Design review of the part built by this model. Coordinates are the model's own, in mm. A direction names the side the tool comes from. Give positions to 0.01 mm unless a question says otherwise; leave off trailing zeros. Loops run counter-clockwise (first coordinate to the right, second up) from the corner with the lowest first, then second, coordinate; pieces in that order, holes last. Notation, with made-up numbers: (63, -22) - (112, -22) arc R31 ccw to (112, 16) - close; hole circle Ø11 at (81, 79). An arc over 180 degrees is marked (long way). Write each question's results on one line, items separated by ' | '.
```python
from build123d import *

# Parameters (mm, degrees)
SKETCH1_W                       = 533.4
SKETCH1_H                       = 2413
BOSS_EXTRUDE1_DEPTH             = 6.35
F_5_16_0_3125_DIAMETER_HOLE1_D  = 7.9375
F_1_4_0_25_DIAMETER_SLOT1_DEPTH = 6.35


# Read off the part's stored shape, not the designer's step: 1/4 (0.25) Diameter Slot1
with BuildPart() as part:
    # Sketch1 → Boss-Extrude1 (new body)
    with BuildSketch(Plane.XY):
        with Locations((0, 1206.5)):
            Rectangle(SKETCH1_W, SKETCH1_H)
        with BuildLine():
            Line((-101.6, 797.56), (101.6, 797.56))
            Line((101.6, 797.56), (101.6, 663.332045059))
            ThreePointArc((101.6, 663.332045059), (209.55, 480.06), (101.6, 296.787954941))
            Line((101.6, 296.787954941), (101.6, 162.56))
            Line((101.6, 162.56), (-101.6, 162.56))
            Line((-101.6, 162.56), (-101.6, 296.787954941))
            ThreePointArc((-101.6, 296.787954941), (-209.55, 480.06), (-101.6, 663.332045059))
            Line((-101.6, 663.332045059), (-101.6, 797.56))
        make_face(mode=Mode.SUBTRACT)
        with BuildLine():
            Line((-101.6, 1508.76), (-101.6, 1374.532045059))
            ThreePointArc((-101.6, 1374.532045059), (-209.55, 1191.26), (-101.6, 1007.987954941))
            Line((-101.6, 1007.987954941), (-101.6, 873.76))
            Line((-101.6, 873.76), (101.6, 873.76))
            Line((101.6, 873.76), (101.6, 1007.987954941))
            ThreePointArc((101.6, 1007.987954941), (209.55, 1191.26), (101.6, 1374.532045059))
            Line((101.6, 1374.532045059), (101.6, 1508.76))
            Line((101.6, 1508.76), (-101.6, 1508.76))
        make_face(mode=Mode.SUBTRACT)
        with BuildLine():
            Line((-101.6, 2219.96), (-101.6, 2085.732045059))
            ThreePointArc((-101.6, 2085.732045059), (-209.55, 1902.46), (-101.6, 1719.187954941))
            Line((-101.6, 1719.187954941), (-101.6, 1584.96))
            Line((-101.6, 1584.96), (101.6, 1584.96))
            Line((101.6, 1584.96), (101.6, 1719.187954941))
            ThreePointArc((101.6, 1719.187954941), (209.55, 1902.46), (101.6, 2085.732045059))
            Line((101.6, 2085.732045059), (101.6, 2219.96))
            Line((101.6, 2219.96), (-101.6, 2219.96))
        make_face(mode=Mode.SUBTRACT)
    extrude(amount=BOSS_EXTRUDE1_DEPTH)

    # 5/16 (0.3125) Diameter Hole1 (through all)
    with Locations(Plane.XY.offset(6.35)):
        with Locations((-76.2, 146.685), (-76.2, 102.235), (-228.6, 177.8), (76.2, 102.235), (76.2, 146.685), (-76.2, 857.885), (-76.2, 813.435), (76.2, 813.435), (76.2, 857.885), (-76.2, 1569.085), (-76.2, 1524.635), (76.2, 1524.635), (76.2, 1569.085), (-76.2, 2280.285), (-76.2, 2235.835), (76.2, 2235.835), (76.2, 2280.285), (228.6, 177.8), (-228.6, 889), (228.6, 889), (-228.6, 1600.2), (228.6, 1600.2), (-228.6, 2311.4), (228.6, 2311.4)):
            Hole(F_5_16_0_3125_DIAMETER_HOLE1_D / 2)

    # 1/4 (0.25) Diameter Slot1 outline → 1/4 (0.25) Diameter Slot1 (cut)
    with BuildSketch(Plane.XY):
        with BuildLine():
            Line((135.8265, 2182.569545059), (135.8265, 2122.244545059))
            ThreePointArc((135.8265, 2122.244545059), (139.0015, 2119.069545059), (142.1765, 2122.244545059))
            Line((142.1765, 2122.244545059), (142.1765, 2182.569545059))
            ThreePointArc((142.1765, 2182.569545059), (139.0015, 2185.744545059), (135.8265, 2182.569545059))
        make_face()
        with BuildLine():
            Line((142.1765, 1411.044545059), (142.1765, 1471.369545059))
            ThreePointArc((142.1765, 1471.369545059), (139.0015, 1474.544545059), (135.8265, 1471.369545059))
            Line((135.8265, 1471.369545059), (135.8265, 1411.044545059))
            ThreePointArc((135.8265, 1411.044545059), (139.0015, 1407.869545059), (142.1765, 1411.044545059))
        make_face()
        with BuildLine():
            Line((142.1765, 699.844545059), (142.1765, 760.169545059))
            ThreePointArc((142.1765, 760.169545059), (139.0015, 763.344545059), (135.8265, 760.169545059))
            Line((135.8265, 760.169545059), (135.8265, 699.844545059))
            ThreePointArc((135.8265, 699.844545059), (139.0015, 696.669545059), (142.1765, 699.844545059))
        make_face()
        with BuildLine():
            Line((-142.1765, 2182.569545059), (-142.1765, 2122.244545059))
            ThreePointArc((-142.1765, 2122.244545059), (-139.0015, 2119.069545059), (-135.8265, 2122.244545059))
            Line((-135.8265, 2122.244545059), (-135.8265, 2182.569545059))
            ThreePointArc((-135.8265, 2182.569545059), (-139.0015, 2185.744545059), (-142.1765, 2182.569545059))
        make_face()
        with BuildLine():
            Line((-135.8265, 1411.044545059), (-135.8265, 1471.369545059))
            ThreePointArc((-135.8265, 1471.369545059), (-139.0015, 1474.544545059), (-142.1765, 1471.369545059))
            Line((-142.1765, 1471.369545059), (-142.1765, 1411.044545059))
            ThreePointArc((-142.1765, 1411.044545059), (-139.0015, 1407.869545059), (-135.8265, 1411.044545059))
        make_face()
        with BuildLine():
            Line((-135.8265, 699.844545059), (-135.8265, 760.169545059))
            ThreePointArc((-135.8265, 760.169545059), (-139.0015, 763.344545059), (-142.1765, 760.169545059))
            Line((-142.1765, 760.169545059), (-142.1765, 699.844545059))
            ThreePointArc((-142.1765, 699.844545059), (-139.0015, 696.669545059), (-135.8265, 699.844545059))
        make_face()
    extrude(amount=F_1_4_0_25_DIAMETER_SLOT1_DEPTH, mode=Mode.SUBTRACT)


solid = part.part
```
Item 1: We need section C-C on y = 1839. Give the boundary of the cut face in (x, z), then the cut area to 3 significant figures.
Output values:
outline: (-266.7, 0) - (-199.71, 0) - (-199.71, 6.35) - (-266.7, 6.35) - close; (199.71, 0) - (266.7, 0) - (266.7, 6.35) - (199.71, 6.35) - close | area: 851 mm²
Item 2: We need section B-B on y = 963. Give the boundary of the cut face in (x, z), then the cut area to 3 significant figures.
Output values:
outline: (-266.7, 0) - (-101.6, 0) - (-101.6, 6.35) - (-266.7, 6.35) - close; (101.6, 0) - (266.7, 0) - (266.7, 6.35) - (101.6, 6.35) - close | area: 2,100 mm²
Item 3: We need section D-D on z = 1.75. Give the number of separate pieces and of enclosed holes in the cut face, then the cut area to 3 significant figures.
Output values:
separate pieces: 1 | enclosed holes: 33 | area: 728,000 mm²
Item 4: We need section A-A on x = -1.5. Give the boundary of the cut face in (y, z).
Output values:
outline: (0, 0) - (162.56, 0) - (162.56, 6.35) - (0, 6.35) - close; (797.56, 0) - (873.76, 0) - (873.76, 6.35) - (797.56, 6.35) - close; (1508.76, 0) - (1584.96, 0) - (1584.96, 6.35) - (1508.76, 6.35) - close; (2219.96, 0) - (2413, 0) - (2413, 6.35) - (2219.96, 6.35) - close
Item 5: Tool access review of faces 1 (the face through (-209.527, 476.937, 3.131)), 2 (the face through (233, 1223, 6.35)): name each direction out of +Z, -Z, +X, -X, +Y, -Y from which nothing blocks a thin tool from reaching the whole face with its end or side.
Output values:
face 1: +Z, -Z | face 2: +Z, +X, -X, +Y, -Y
Item 6: Draft analysis for pull direction X (two halves, no side actions). For faces 3 (the face through (-209.527, 1905.583, 3.131)), 4 (the face through (233, 1223, 0)), state which applies: +X half, -X half, draft (parallel to the pull), parting line (faces both ways), or undercut.
Output values:
face 3: undercut | face 4: draft
Item 7: Wall thickness on probe 1 along Y at (x, z) = (-228.6, 2.25); probe 2 along Y at (x, z) = (96.5, 6); probe 3 along X at (y, z) = (2311.4, 4.5): over which ranges is each line inside the solid? List them lowest first.
Output values:
probe 1: y = 0 to 173.83, 181.77 to 885.03, 892.97 to 1596.23, 1604.17 to 2307.43, 2315.37 to 2413 | probe 2: y = 0 to 162.56, 797.56 to 873.76, 1508.76 to 1584.96, 2219.96 to 2413 | probe 3: x = -266.7 to -232.57, -224.63 to 224.63, 232.57 to 266.7
